For this review, take the finished solid that the model builds, in its own axes (mm). Face numbers are marked on the shaded views. A direction names the side the tool comes from. Round coordinates to 2 decimals unless told otherwise and drop trailing zeros. Order: outer loops, then holes, each group sorted by start corner. A loop starts at its lowest first (then second) coordinate and runs counter-clockwise, first axis right, second up. Notation, with made-up numbers: M -38.5,-17.75 L 2.5,-17.75 A10 ccw 2.5,-2.75 Z; hole C -40,30.5 d11. An arc over 180 degrees is marked long. Answer as a JSON object with one key per item and string values.
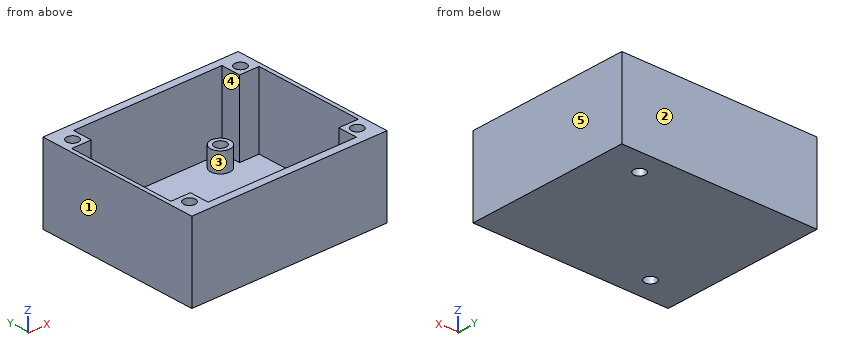
from build123d import *

# Parameters (mm, degrees)
F0_W      = 50
F0_H      = 42
F1_DEPTH  = 20
F2_W      = 38
F2_H      = 38
F3_DEPTH  = 19
F4_W      = 5
F4_H      = 38
F5_DEPTH  = 19
F6_W      = 5
F6_H      = 5
F7_DEPTH  = 19
F8_R      = 1.5
F9_DEPTH  = 10
F10_R     = 2.5
F10_R_2   = 1.5
F11_DEPTH = 5
F12_DEPTH = 1


with BuildPart() as f1:
    # F0 (on Top) → F1 (new body)
    with BuildSketch(Plane.XY):
        with Locations((-37.0541260391, 42.2422697991)):
            Rectangle(F0_W, F0_H)
    extrude(amount=F1_DEPTH)

    # F2 (on face) → F3 (cut)
    with BuildSketch(Plane.XY.offset(20)):
        with Locations((-37.0541260391, 42.2422697991)):
            Rectangle(F2_W, F2_H)
    extrude(amount=-F3_DEPTH, mode=Mode.SUBTRACT)

    # F4 (on face) → F5 (cut)
    with BuildSketch(Plane.XY.offset(20)):
        with Locations((-15.5541260391, 42.2422697991)):
            Rectangle(F4_W, F4_H)
        with Locations((-58.5541260391, 42.2422697991)):
            Rectangle(F4_W, F4_H)
    extrude(amount=-F5_DEPTH, mode=Mode.SUBTRACT)

    # F6 (on face) → F7 (join)
    with BuildSketch(Plane.XY.offset(1)):
        with Locations((-15.5541260391, 58.7422697991)):
            Rectangle(F6_W, F6_H)
        with Locations((-15.5541260391, 25.7422697991)):
            Rectangle(F6_W, F6_H)
        with Locations((-58.5541260391, 58.7422697991)):
            Rectangle(F6_W, F6_H)
        with Locations((-58.5541260391, 25.7422697991)):
            Rectangle(F6_W, F6_H)
    extrude(amount=F7_DEPTH)

    # F8 (on face) → F9 (cut)
    with BuildSketch(Plane.XY.offset(20)):
        with Locations((-15.5541260391, 58.7422697991)):
            Circle(F8_R)
        with Locations((-15.5541260391, 25.7422697991)):
            Circle(F8_R)
        with Locations((-58.5541260391, 25.7422697991)):
            Circle(F8_R)
        with Locations((-58.5541260391, 58.7422697991)):
            Circle(F8_R)
    extrude(amount=-F9_DEPTH, mode=Mode.SUBTRACT)

    # F10 (on face) → F11 (join)
    with BuildSketch(Plane.XY.offset(1)):
        with Locations((-22.0541260391, 57.2422697991)):
            Circle(F10_R)
        with Locations((-22.0541260391, 57.2422697991)):
            Circle(F10_R_2, mode=Mode.SUBTRACT)
        with Locations((-52.0541260391, 27.2422697991)):
            Circle(F10_R)
        with Locations((-52.0541260391, 27.2422697991)):
            Circle(F10_R_2, mode=Mode.SUBTRACT)
    extrude(amount=F11_DEPTH)

    # F12 (cut): faces of the model
    f12_faces = [f1.faces().sort_by_distance(p)[0] for p in [
        (-22.0541260391, 57.2422697991, 1),
        (-52.0541260391, 27.2422697991, 1),
    ]]
    extrude(f12_faces, amount=-F12_DEPTH, mode=Mode.SUBTRACT)


solid = f1.part
1) Add section B-B on x = -21.5. State the section outline as (y, z) points.
Geometry check:
{"outline": "M 21.24,0 L 55.85,0 L 55.85,6 L 54.8,6 L 54.8,1 L 23.24,1 L 23.24,20 L 21.24,20 Z; M 58.64,0 L 63.24,0 L 63.24,20 L 61.24,20 L 61.24,1 L 59.68,1 L 59.68,6 L 58.64,6 Z"}
2) Mouldability with a two-part tool opening along Y and no side actions: class the marked faces 1, 2 and 3 as +Y half, -Y half, draft (parallel to the pull), parting line (faces both ways), or undercut.
Geometry check:
{"face 1": "draft", "face 2": "+Y half", "face 3": "undercut"}
3) Machinability: for the marked faces 4 and 5, which of the approach directions +Z, -Z, +X, -X, +Y, -Y give a long, thin tool a straight path to every point of the face, cutting with its end or side? Answer none if there is none.
Geometry check:
{"face 4": "+Z", "face 5": "+Z, -Z, +X, +Y, -Y"}
4) For L1, parallel to X at y = 51, z = 12.25; L2, parallel to Y at x = -50, z = 16.5; L3, parallel to X at y = 60, z = 11.25, list the stretches that pass through material, from the lowest coordinate up.
Geometry check:
{"L1": "x = -62.05 to -61.05, -13.05 to -12.05", "L2": "y = 21.24 to 23.24, 61.24 to 63.24", "L3": "x = -62.05 to -59.37, -57.74 to -56.05, -18.05 to -16.37, -14.74 to -12.05"}
5) Insertion check: P1, Ø1.5, axis at x = -21, y = 57.5, coming from the +Z side; P2, Ø1.5, axis at x = -35, y = 34, coming from the +Z side. Each pin has a flat end and moves straight along its axis. Give the tip position at first contact, or say it passes through.
Geometry check:
{"P1": "stops at z = 6", "P2": "stops at z = 1"}
6) Add section D-D on z = 16. State the section outline as (x, y) points, and give its area (3 significant figures).
Geometry check:
{"outline": "M -62.05,21.24 L -12.05,21.24 L -12.05,63.24 L -62.05,63.24 Z; hole M -61.05,28.24 L -56.05,28.24 L -56.05,23.24 L -18.05,23.24 L -18.05,28.24 L -13.05,28.24 L -13.05,56.24 L -18.05,56.24 L -18.05,61.24 L -56.05,61.24 L -56.05,56.24 L -61.05,56.24 Z; hole C -58.55,25.74 d3; hole C -58.55,58.74 d3; hole C -15.55,25.74 d3; hole C -15.55,58.74 d3", "area": "348 mm²"}
7) Add section C-C on y = 38. State the section outline as (x, z) points.
Geometry check:
{"outline": "M -62.05,0 L -12.05,0 L -12.05,20 L -13.05,20 L -13.05,1 L -61.05,1 L -61.05,20 L -62.05,20 Z"}
8) Add section A-A on z = 3. State the section outline as (x, y) points.
Geometry check:
{"outline": "M -62.05,21.24 L -12.05,21.24 L -12.05,63.24 L -62.05,63.24 Z; C -52.05,27.24 d5; C -22.05,57.24 d5; hole M -61.05,28.24 L -56.05,28.24 L -56.05,23.24 L -18.05,23.24 L -18.05,28.24 L -13.05,28.24 L -13.05,56.24 L -18.05,56.24 L -18.05,61.24 L -56.05,61.24 L -56.05,56.24 L -61.05,56.24 Z; hole C -52.05,27.24 d3; hole C -22.05,57.24 d3"}
